The listing builds one solid part. Answer for the finished solid, in the listing's coordinates (mm). Face numbers are marked on the shaded views. A direction names the side the tool comes from. Give positions to 0.01 mm unless a question says otherwise; leave off trailing zeros. Write each loop counter-clockwise with the first axis right and the second up, starting at its lowest first coordinate (ties: lowest second). Pieces come first, ordered by that corner, then holes. Notation, with made-up numbers: (80.25, -3.75) - (132.25, -3.75) arc R26 cw to (132.25, 33.25) - close; hole circle Ø3 at (12, 37). An arc over 180 degrees is marked (long way). Answer in a Markdown table with one row per item. Add a question column.
from build123d import *

# Parameters (mm, degrees)
SKETCH1_R           = 2.4
BOSS_EXTRUDE1_DEPTH = 10
SKETCH2_R           = 4.25
BOSS_EXTRUDE2_DEPTH = 5
CUT_EXTRUDE1_DEPTH  = 3
CHAMFER1_SIZE       = 0.5
FILLET1_R           = 0.5


with BuildPart() as part:
    # Sketch1 → Boss-Extrude1 (new body)
    with BuildSketch(Plane(origin=(0, 0, 0), x_dir=(1, 0, 0), z_dir=(0, 1, 0))):
        with Locations(Location((0, 0, 0), (0, 0, 270))):
            Circle(SKETCH1_R)
    extrude(amount=BOSS_EXTRUDE1_DEPTH)

    # Sketch2 → Boss-Extrude2 (add)
    with BuildSketch(Plane(origin=(0, 10, 0), x_dir=(1, 0, 0), z_dir=(0, 1, 0))):
        with Locations(Location((0, 0, 0), (0, 0, 270))):
            Circle(SKETCH2_R)
    extrude(amount=BOSS_EXTRUDE2_DEPTH)

    # Sketch3 → Cut-Extrude1 (cut)
    with BuildSketch(Plane(origin=(0, 15, 0), x_dir=(1, 0, 0), z_dir=(0, 1, 0))):
        with BuildLine():
            Line((2.165063509, 0.25), (1.299038106, 1.75))
            ThreePointArc((1.299038106, 1.75), (1.116025404, 1.933012702), (0.866025404, 2))
            Line((0.866025404, 2), (-0.866025404, 2))
            ThreePointArc((-0.866025404, 2), (-1.116025404, 1.933012702), (-1.299038106, 1.75))
            Line((-1.299038106, 1.75), (-2.165063509, 0.25))
            ThreePointArc((-2.165063509, 0.25), (-2.232050808, 0), (-2.165063509, -0.25))
            Line((-2.165063509, -0.25), (-1.299038106, -1.75))
            ThreePointArc((-1.299038106, -1.75), (-1.116025404, -1.933012702), (-0.866025404, -2))
            Line((-0.866025404, -2), (0.866025404, -2))
            ThreePointArc((0.866025404, -2), (1.116025404, -1.933012702), (1.299038106, -1.75))
            Line((1.299038106, -1.75), (2.165063509, -0.25))
            ThreePointArc((2.165063509, -0.25), (2.232050808, 0), (2.165063509, 0.25))
        make_face()
    extrude(amount=-CUT_EXTRUDE1_DEPTH, mode=Mode.SUBTRACT)

    # Chamfer1
    chamfer1_edges = [part.edges().sort_by_distance(p)[0] for p in [
        (-2.232050808, 12, 0),
        (-1.732050808, 12, -1),
        (-1.116025404, 12, -1.933012702),
        (0, 12, -2),
        (1.116025404, 12, -1.933012702),
        (1.732050808, 12, -1),
        (2.232050808, 12, 0),
        (1.732050808, 12, 1),
        (1.116025404, 12, 1.933012702),
        (0, 12, 2),
        (-1.116025404, 12, 1.933012702),
        (-1.732050808, 12, 1),
        (-2.232050808, 15, 0),
        (-1.732050808, 15, 1),
        (-1.116025404, 15, 1.933012702),
        (0, 15, 2),
        (1.116025404, 15, 1.933012702),
        (1.732050808, 15, 1),
        (2.232050808, 15, 0),
        (1.732050808, 15, -1),
        (1.116025404, 15, -1.933012702),
        (0, 15, -2),
        (-1.116025404, 15, -1.933012702),
        (-1.732050808, 15, -1),
    ]]
    chamfer(chamfer1_edges, length=CHAMFER1_SIZE - 0.0001)  # a hair under: the kernel refuses the full size

    # Fillet1
    fillet1_edges = [part.edges().sort_by_distance(p)[0] for p in [
        (0, 15, -4.25),
    ]]
    fillet(fillet1_edges, radius=FILLET1_R)


solid = part.part
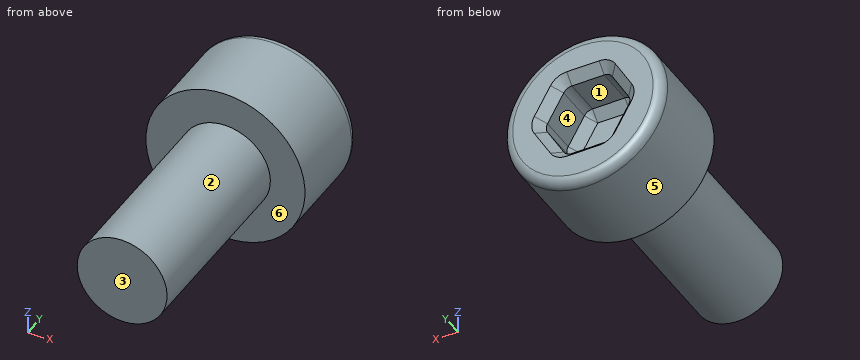
1. Section B-B (y = 3.75) is taken. Give the vertices of the cut face in (x, z).
2. A tool of negligible diameter and unlimited length cuts with its end or side. For the marked faces 4, 5 and 6, from which of +Z, -Z, +X, -X, +Y, -Y can it reach the whole face along a straight path? Write none if from no direction.
3. Section A-A (x = 0) is taken. Give the vertices of the cut face in (y, z).
4. Given pin 1 Ø3.5 at (x, z) = (0.5, 0.5) entering from +Y; pin 2 Ø3 at (x, y) = (1.5, 7.5) entering from +Z; pin 3 Ø1 at (x, y) = (3, 6) entering from +Z; pin 4 Ø4 at (y, z) = (4, -2) entering from +X, each flat-ended and moving along its own axis, determine where each tip first touches the part or whether it passes through.
5. The mould has two halves that part along Z. Classify the marked faces 1, 2 and 3: +Z half, -Z half, draft (parallel to the pull), parting line (faces both ways), or undercut.
6. Straight lines are drawn through the part: L1, parallel to Y at x = 2.5, z = -1; L2, parallel to X at y = 13.75, z = -0.75; L3, parallel to Z at x = 0.75, y = 5. For each, find the intervals that lie inside material, in ascending order. Write a range as [from, to].
Geometry check:
| question | item | result |
|---|---|---|
| 1 | outline | circle Ø4.8 at (0, 0) |
| 2 | face 4 | +Y |
| 2 | face 5 | +Y, -Y |
| 2 | face 6 | -Y |
| 3 | outline | (0, -2.4) - (10, -2.4) - (10, -4.25) - (14.5, -4.25) arc R0.5 ccw to (15, -3.75) - (15, -2.5) - (14.5, -2) - (12.5, -2) - (12, -1.5) - (12, 1.5) - (12.5, 2) - (14.5, 2) - (15, 2.5) - (15, 3.75) arc R0.5 ccw to (14.5, 4.25) - (10, 4.25) - (10, 2.4) - (0, 2.4) - close |
| 4 | pin 1 | y = 14.93 |
| 4 | pin 2 | z = 2.4 |
| 4 | pin 3 | through |
| 4 | pin 4 | x = 2.4 |
| 5 | face 1 | undercut |
| 5 | face 2 | parting line |
| 5 | face 3 | draft |
| 6 | L1 | [10, 15] |
| 6 | L2 | [-4.18, -1.88], [1.88, 4.18] |
| 6 | L3 | [-2.28, 2.28] |
